Could you check a few things on this model? Use its own coordinates, in mm. A direction names the side the tool comes from. Coordinates: 2 decimals unless noted, no trailing zeros. Write each loop counter-clockwise with the first axis right and the second up, starting at its lowest first coordinate (ties: lowest second). Pieces come first, ordered by that corner, then holes.
```python
from build123d import *

# Parameters (mm, degrees)
BOSS_EXTRUDE1_DEPTH   = 3.175
FILLET1_R             = 3.175
F_6_CLEARANCE_HOLE1_D = 4.3053
F_2_CLEARANCE_HOLE1_D = 2.7051
FILLET2_R             = 12.7


with BuildPart() as part:
    # Sketch1 → Boss-Extrude1 (new body)
    with BuildSketch(Plane.XY):
        with BuildLine():
            Line((-0.394361249, -4.746144273), (24.410778081, -6.807224837))
            Line((24.410778081, -6.807224837), (67.367437597, -24.620374852))
            ThreePointArc((67.367437597, -24.620374852), (67.932057441, -24.79496394), (68.519252784, -24.861885891))
            Line((68.519252784, -24.861885891), (86.557178011, -25.22763618))
            ThreePointArc((86.557178011, -25.22763618), (90.731319104, -22.926733092), (90.821358826, -18.161284348))
            Line((90.821358826, -18.161284348), (80.17216718, 1.094759821))
            ThreePointArc((80.17216718, 1.094759821), (79.70833798, 1.731518351), (79.102014267, 2.234480087))
            Line((79.102014267, 2.234480087), (36.315798025, 29.544973103))
            ThreePointArc((36.315798025, 29.544973103), (31.002904726, 29.418519327), (29.114914109, 24.450791758))
            Line((29.114914109, 24.450791758), (30.886207986, 16.841662569))
            Line((30.886207986, 16.841662569), (-1.692935369, 4.451446516))
            ThreePointArc((-1.692935369, 4.451446516), (-4.715731213, -0.6657968), (-0.394361249, -4.746144273))
        make_face()
        Polygon((72.732635266, -19.970882517), (23.451745327, 0.464782063), (29.829511311, 15.844853618), (79.11040125, -4.590810962), align=None, mode=Mode.SUBTRACT)
    extrude(amount=BOSS_EXTRUDE1_DEPTH)

    # Fillet1
    fillet1_edges = [part.edges().sort_by_distance(p)[0] for p in [
        (72.732635266, -19.970882517, 1.5875),
        (79.11040125, -4.590810962, 1.5875),
        (29.829511311, 15.844853618, 1.5875),
        (23.451745327, 0.464782063, 1.5875),
    ]]
    fillet(fillet1_edges, radius=FILLET1_R)

    # #6 Clearance Hole1 (through all)
    with Locations(Plane.XY.offset(3.175)):
        with Locations((0, 0), (33.7533947, 25.530562131), (86.653726131, -20.46611492)):
            Hole(F_6_CLEARANCE_HOLE1_D / 2)

    # #2 Clearance Hole1 (through all)
    with Locations(Plane.XY.offset(3.175)):
        with Locations((33.97852838, 17.561509485), (77.393745383, -0.441793894), (68.583618198, -21.687538385), (25.168401194, -3.684235006)):
            Hole(F_2_CLEARANCE_HOLE1_D / 2)

    # Fillet2
    fillet2_edges = [part.edges().sort_by_distance(p)[0] for p in [
        (24.410778081, -6.807224837, 1.5875),
        (30.886207986, 16.841662569, 1.5875),
    ]]
    fillet(fillet2_edges, radius=FILLET2_R)


solid = part.part
```
1. I want a section at A-A on x = 38. Please give me the cut outline in (y, z) (3 decimals).
Verdict:
outline: (-12.442, 0) - (-5.568, 0) - (-5.568, 3.175) - (-12.442, 3.175) - close; (12.457, 0) - (28.47, 0) - (28.47, 3.175) - (12.457, 3.175) - close
2. On a 3-axis mill with a long thin cutter (end or side, diameter ignored), from which of +Z, -Z, +X, -X, +Y, -Y can I reach the whole of each face in a straight line? I mean faces 1 (the face through (48.4, -9.88, 1.57)), 2 (the face through (10.86, -5.68, 1.57)). Say none if no direction works.
Verdict:
face 1: +Z, -Z
face 2: +Z, -Z, -X, -Y
3. Please list where these lines run through material, in increasing order: line 1 along Y through (x, z) = (77, 1.95); line 2 along Y through (x, z) = (68, 2.25); line 3 along X through (y, z) = (-10, 2.6).
Verdict:
line 1: y = -25.03 to -9.68, -3.87 to -1.74, 0.85 to 3.58
line 2: y = -24.81 to -22.91, -20.47 to -18.01, 0.02 to 9.32
line 3: x = 32.11 to 48.69, 76.87 to 86.31
4. I want a section at C-C on x = 82. Please give me the cut outline in (y, z) (3 decimals), plus the area to 3 significant figures.
Verdict:
outline: (-25.135, 0) - (-2.21, 0) - (-2.21, 3.175) - (-25.135, 3.175) - close
area: 72.8 mm2
5. If we mould it in two halves opening along Y, with no side actions, what happens to faces 3 (the face through (9.72, 8.79, 1.57)), 4 (the face through (46.518, -15.975, 1.565)), 5 (the face through (47, 11, 0)), 6 (the face through (77.91, -5.13, 1.61))? For each: pulls with the +Y half, pulls with the -Y half, needs draft (parallel to the pull), parting line crosses it, or undercut.
Verdict:
face 3: pulls with the +Y half
face 4: pulls with the -Y half
face 5: needs draft
face 6: undercut
6. I want a section at B-B on z = 2.55. Give the number of separate pieces and of enclosed holes in the cut face, plus the area to 3 significant figures.
Verdict:
separate pieces: 1
enclosed holes: 8
area: 1,620 mm2
7. For pin 1 (5 mm diameter, centred on x = 33.75, y = 25.53, fed in from +Z) (3 decimals); pin 2 (1.6 mm diameter, centred on x = 77.39, y = -0.44, fed in from +Z), each with a flat end and sliding along its axis, tell me the tip position at first contact or that it passes through.
Verdict:
pin 1: stops at z = 3.175
pin 2: passes through
